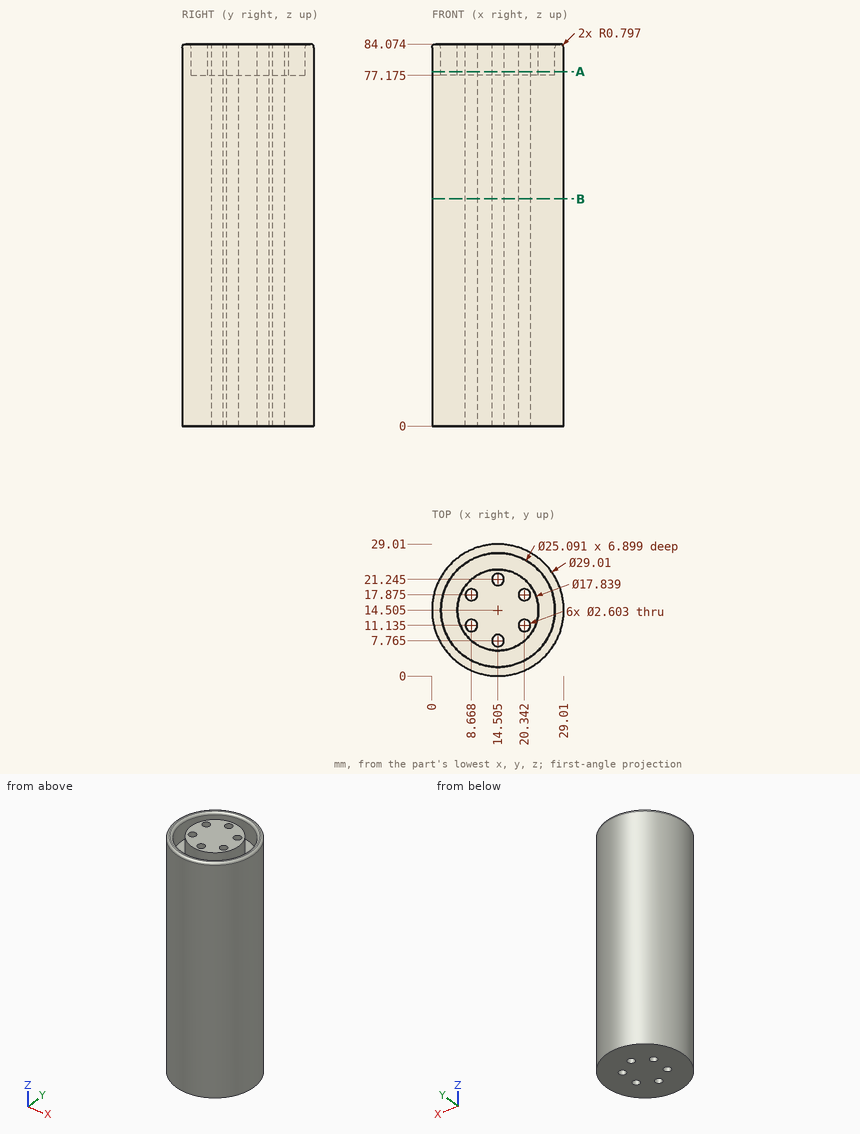
Geometry: see drawing. Coordinates: mm, zero at the bounding-box minimum. Round coordinates to 2 decimals unless told otherwise and drop trailing zeros. Loops run counter-clockwise (first coordinate to the right, second up) from the corner with the lowest first, then second, coordinate; pieces in that order, holes last. Notation, with made-up numbers: (56, -3.75) - (105, -3.75) arc R21 ccw to (105, 21.25) - close; hole circle Ø8 at (35.5, 57). An arc over 180 degrees is marked (long way). Use CSV: the item, a comma, the result in double quotes.
Q1. Section query B-B, the plane z = 50. Output: boundary loops of the cut face in (x, y) (1 decimal).
Reported:
outline,"circle Ø29 at (14.5, 14.5); hole circle Ø2.6 at (8.7, 11.1); hole circle Ø2.6 at (8.7, 17.9); hole circle Ø2.6 at (14.5, 7.8); hole circle Ø2.6 at (14.5, 21.2); hole circle Ø2.6 at (20.3, 11.1); hole circle Ø2.6 at (20.3, 17.9)"
Q2. Ray query, line 1 along X through (y, z) = (19, 58) (1 decimal); line 2 along Y through (x, z) = (9.25, 9) (1 decimal); line 3 along Y through (x, z) = (20.25, 10) (1 decimal). Return the intervals inside material, ascending.
Reported:
line 1,"0.7 to 8, 9.3 to 19.7, 21 to 28.3"
line 2,"1 to 10, 12.3 to 16.7, 19 to 28"
line 3,"1.2 to 9.8, 12.4 to 16.6, 19.2 to 27.8"
Q3. Section query A-A, the plane z = 78. Give the number of separate pieces and of enclosed holes in the cut face.
Reported:
separate pieces,"2"
enclosed holes,"7"
Q4. Pin query (flat end, axial travel): pin 1 Ø10 at (x, z) = (15.5, 14) entering from +Y; pin 2 Ø12 at (y, z) = (24.5, 44) entering from +X; pin 3 Ø6 at (x, z) = (26, 47.5) entering from -Y; pin 4 Ø8 at (x, z) = (3, 39) entering from -Y. Return the tip coordinate at first contact, or that it passes through.
Reported:
pin 1,"y = 29.01"
pin 2,"x = 28.45"
pin 3,"y = 2.75"
pin 4,"y = 2.09"
